```python
from build123d import *

# Parameters (mm, degrees)
SECSKE_W      = 1.4
SECSKE_H      = 9.5
EXTCUT_DEPTH  = 25.788303693
EXTCUTS_COUNT = 16
EXTCUTS_ANGLE = 337.5
INTCUT_DEPTH  = 25.565286833
INTCUTS_COUNT = 12
INTCUTS_ANGLE = 330


with BuildPart() as part:
    # SecSke → Body (revolve)
    with BuildSketch(Plane.XY, mode=Mode.PRIVATE) as body_sk:
        with Locations((-0.7, 12.75)):
            Rectangle(SECSKE_W, SECSKE_H)
    revolve(body_sk.sketch.rotate(Axis((-34.925, 0, 0), (1, 0, 0)), 90), axis=Axis((-34.925, 0, 0), (1, 0, 0)))

    # ExtCutSke → ExtCut (cut, through all)
    with BuildSketch(Plane(origin=(0, 0, 0), x_dir=(0, 0, -1), z_dir=(1, 0, 0))):
        with BuildLine():
            Line((-2.696172468, 18.176118371), (-0.80653001, 13.67623886))
            ThreePointArc((-0.80653001, 13.67623886), (0, 13.7), (0.80653001, 13.67623886))
            Line((0.80653001, 13.67623886), (2.696172468, 18.176118371))
            ThreePointArc((2.696172468, 18.176118371), (0, 18.375), (-2.696172468, 18.176118371))
        make_face()
    extcut = extrude(amount=-EXTCUT_DEPTH, mode=Mode.SUBTRACT)

    # ExtCuts: ExtCut ×16 about axis
    extcuts_axis = Axis((-34.925, 0, 0), (1, 0, 0))
    for i in range(1, EXTCUTS_COUNT):
        add(extcut.rotate(extcuts_axis, i * EXTCUTS_ANGLE / (EXTCUTS_COUNT - 1)), mode=Mode.SUBTRACT)

    # IntCutSke → IntCut (cut, through all)
    with BuildSketch(Plane(origin=(0, 0, 0), x_dir=(0, 0, -1), z_dir=(1, 0, 0))):
        with BuildLine():
            Line((-0.697197358, 10.637176122), (-1.326257139, 7.483384395))
            ThreePointArc((-1.326257139, 7.483384395), (0, 7.6), (1.326257139, 7.483384395))
            Line((1.326257139, 7.483384395), (0.697197358, 10.637176122))
            ThreePointArc((0.697197358, 10.637176122), (0, 10.66), (-0.697197358, 10.637176122))
        make_face()
    intcut = extrude(amount=-INTCUT_DEPTH, mode=Mode.SUBTRACT)

    # IntCuts: IntCut ×12 about axis
    intcuts_axis = Axis((-34.925, 0, 0), (1, 0, 0))
    for i in range(1, INTCUTS_COUNT):
        add(intcut.rotate(intcuts_axis, i * INTCUTS_ANGLE / (INTCUTS_COUNT - 1)), mode=Mode.SUBTRACT)


solid = part.part
```
Geometry check sheet. Reference: the model listing, model coordinates, mm. A direction names the side the tool comes from. Coordinates: 2 decimals unless noted, no trailing zeros. Order: outer loops, then holes, each group sorted by start corner. A loop starts at its lowest first (then second) coordinate and runs counter-clockwise, first axis right, second up. Notation, with made-up numbers: (-28, 61) - (7, 61) arc R36 cw to (7, 96) - close; hole circle Ø11 at (30, -36.5). An arc over 180 degrees is marked (long way). Answer in a Markdown table with one row per item. Add a question column.
1. Material ranges on L1, parallel to Z at x = -1.3, y = -13; L2, parallel to Y at x = -0.7, z = 10.5; L3, parallel to Y at x = -0.3, z = 15, recorded low to high. Write a range as [from, to].
2. Section check A-A (z = 0). Enter the section's corners in (x, y).
3. Section check C-C (y = -11.5). Enter the section's corners in (x, z), plus the area to 3 significant figures.
4. Section check B-B (y = 3.5). Enter the section's corners in (x, z).
5. Draft check along Z on faces 4 (the face through (-0.69, 7.411, -13.745)), 5 (the face through (-0.69, -9.842, 12.055)), 6 (the face through (-0.69, -3.399, 17.167)). Enter one of: +Z half, -Z half, draft (parallel to the pull), parting line (faces both ways), or undercut.
6. Access from +Z, -Z, +X, -X, +Y, -Y to the whole of each face (thin tool, end or side, straight path). Record for faces 1 (the face through (-0.69, -12.653, -5.253)), 2 (the face through (-0.69, 5.648, -5.665)), 3 (the face through (-0.69, 1.565, 15.483)).
Data:
| question | item | result |
|---|---|---|
| 1 | L1 | z = [-10.23, -6.66], [-4.49, 4.49], [6.66, 10.23] |
| 1 | L2 | y = [-14, -13.67], [-9.21, -0.72], [0.72, 9.21], [13.67, 14] |
| 1 | L3 | y = [-9.01, -8.68], [-4.48, -1.36], [1.36, 4.48], [8.68, 9.01] |
| 2 | outline | (-1.4, -13.7) - (0, -13.7) - (0, -10.66) - (-1.4, -10.66) - close; (-1.4, 10.66) - (0, 10.66) - (0, 13.7) - (-1.4, 13.7) - close |
| 3 | outline | (-1.4, -9.61) - (0, -9.61) - (0, 9.61) - (-1.4, 9.61) - close |
| 3 | area | 26.9 mm² |
| 4 | outline | (-1.4, -17.15) - (0, -17.15) - (0, -8.18) - (-1.4, -8.18) - close; (-1.4, 8.18) - (0, 8.18) - (0, 17.15) - (-1.4, 17.15) - close |
| 5 | face 4 | -Z half |
| 5 | face 5 | undercut |
| 5 | face 6 | +Z half |
| 6 | face 1 | +X, -X, -Y |
| 6 | face 2 | +X, -X |
| 6 | face 3 | +Z, +X, -X |
